from build123d import *

# Parameters (mm, degrees)
SKETCH1_R                       = 9.5
BOSS_EXTRUDE1_DEPTH             = 25
BOSS_EXTRUDE2_DEPTH             = 6
BOSS_EXTRUDE2_DEPTH_BACK        = 108
SKETCH2_R                       = 35
BOSS_EXTRUDE3_DEPTH             = 6.5
BOSS_EXTRUDE3_DEPTH_BACK        = 44.5
SKETCH3_R                       = 35
BOSS_EXTRUDE4_DEPTH             = 77
RIB1_REACH                      = 331.39
SKETCH5_WALLS_W                 = 19
SKETCH5_WALLS_H                 = 685.704980613
RIB2_REACH                      = 335.377
SKETCH6_WALLS_W                 = 19
SKETCH6_WALLS_H                 = 696.792690098
F_6_0MM_DOWEL_HOLE1_D           = 6
F_6_0MM_DOWEL_HOLE1_DEPTH       = 54
F_6_0MM_DOWEL_HOLE1_CSINK_D     = 6.05
F_6_0MM_DOWEL_HOLE1_CSINK_ANGLE = 90
F_6_0MM_DOWEL_HOLE1_TIP         = 1.802581857


with BuildPart() as part:
    # Sketch1 → Boss-Extrude1 (new body)
    with BuildSketch(Plane(origin=(0, 0, 0), x_dir=(1, 0, 0), z_dir=(0, 1, 0))):
        with BuildLine():
            Line((0, 102), (0, 0))
            Line((0, 0), (200, 0))
            Line((200, 0), (200, 213))
            Line((200, 213), (166, 213))
            Line((166, 213), (166, 147))
            ThreePointArc((166, 147), (152.819805153, 115.180194847), (121, 102))
            Line((121, 102), (0, 102))
        make_face()
        with Locations(Location((16, 57, 0), (0, 0, 270))):
            Circle(SKETCH1_R, mode=Mode.SUBTRACT)
        with Locations(Location((16, 19, 0), (0, 0, 270))):
            Circle(SKETCH1_R, mode=Mode.SUBTRACT)
        with Locations(Location((168, 19, 0), (0, 0, 270))):
            Circle(SKETCH1_R, mode=Mode.SUBTRACT)
        with Locations(Location((168, 57, 0), (0, 0, 270))):
            Circle(SKETCH1_R, mode=Mode.SUBTRACT)
    extrude(amount=BOSS_EXTRUDE1_DEPTH)



with BuildPart() as body_2:
    # Sketch2 → Boss-Extrude2 (new, two sides: drawn at the far end of the back side and taken through both)
    with BuildSketch(Plane.XY.offset(-BOSS_EXTRUDE2_DEPTH_BACK)):
        with Locations((83, 102)):
            Circle(SKETCH2_R)
    extrude(amount=BOSS_EXTRUDE2_DEPTH + BOSS_EXTRUDE2_DEPTH_BACK)


with BuildPart() as body_3:
    # Sketch3 → Boss-Extrude3 (new, two sides: drawn at the far end of the back side and taken through both)
    with BuildSketch(Plane(origin=(200, 0, 0), x_dir=(0, 0, -1), z_dir=(1, 0, 0)).offset(-BOSS_EXTRUDE3_DEPTH_BACK)):
        with Locations((188, 102)):
            Circle(SKETCH3_R)
    extrude(amount=BOSS_EXTRUDE3_DEPTH + BOSS_EXTRUDE3_DEPTH_BACK)


with BuildPart() as part_1:
    add(part.part)

    add(body_2.part)  # Boss-Extrude4 merges body 2

    add(body_3.part)  # Boss-Extrude4 merges body 3
    # Sketch4 → Boss-Extrude4 (add)
    with BuildSketch(Plane(origin=(0, 25, 0), x_dir=(1, 0, 0), z_dir=(0, 1, 0))):
        with BuildLine():
            Line((121, 102), (48, 102))
            Line((48, 102), (48, 83))
            Line((48, 83), (121, 83))
            ThreePointArc((121, 83), (166.254833996, 101.745166004), (185, 147))
            Line((185, 147), (185, 223))
            Line((185, 223), (166, 223))
            Line((166, 223), (166, 147))
            ThreePointArc((166, 147), (152.819805153, 115.180194847), (121, 102))
        make_face()
    extrude(amount=BOSS_EXTRUDE4_DEPTH)

    # Sketch5 walls → Rib1 (add, up to next)
    with BuildSketch(Plane(origin=(200, 0, 0), x_dir=(0, 0, -1), z_dir=(1, 0, 0)), mode=Mode.PRIVATE) as rib1_sk1:
        with Locations((188, 47.27733831)):
            Rectangle(SKETCH5_WALLS_W, SKETCH5_WALLS_H)
    rib1_tool1 = extrude(rib1_sk1.sketch, amount=-RIB1_REACH, mode=Mode.PRIVATE) - part_1.part
    add(rib1_tool1.solids().sort_by_distance((200, 47.277338311, -188))[0])

    # Sketch6 walls → Rib2 (add, up to next)
    with BuildSketch(Plane.XY, mode=Mode.PRIVATE) as rib2_sk1:
        with Locations((83, 44.133110569)):
            Rectangle(SKETCH6_WALLS_W, SKETCH6_WALLS_H)
    rib2_tool1 = extrude(rib2_sk1.sketch, amount=-RIB2_REACH, mode=Mode.PRIVATE) - part_1.part
    add(rib2_tool1.solids().sort_by_distance((83, 44.133110569, 0))[0])

    # Ø6.0mm Dowel Hole1
    with Locations(Plane(origin=(206.5, 99.319699539, -190.863289795), x_dir=(0, 0, 1), z_dir=(1, 0, 0))):
        with Locations((0, 0)):
            CounterSinkHole(F_6_0MM_DOWEL_HOLE1_D / 2, F_6_0MM_DOWEL_HOLE1_CSINK_D / 2, depth=F_6_0MM_DOWEL_HOLE1_DEPTH, counter_sink_angle=F_6_0MM_DOWEL_HOLE1_CSINK_ANGLE)
            with Locations((0, 0, -(F_6_0MM_DOWEL_HOLE1_DEPTH + F_6_0MM_DOWEL_HOLE1_TIP / 2))):  # 118° drill point
                Cone(0, F_6_0MM_DOWEL_HOLE1_D / 2, F_6_0MM_DOWEL_HOLE1_TIP, mode=Mode.SUBTRACT)


solid = part_1.part
Verification items for the finished model (mm, model axes). A direction names the side the tool comes from. Coordinates: 2 decimals unless noted, no trailing zeros. Loops run counter-clockwise (first coordinate to the right, second up) from the corner with the lowest first, then second, coordinate; pieces in that order, holes last. Notation, with made-up numbers: (86.5, -21) -> (132.5, -21) arc R35 cw to (132.5, 17) -> close; hole circle Ø9 at (5.5, 23.25). An arc over 180 degrees is marked (long way). Answer as a JSON object with one key per item and string values. Group by question number.
Item 1: Sectioned sample at D-D on y = 54. Record the boundary of the cut face in (x, z), plus the area to 3 significant figures.
Item 2: Tool access check on faces 1 (the flat face through (83, 102, -108)), 2 (the cylindrical face through (165.755, 62.961, -101.25)), 3 (the flat face through (183, 12, -213)), 4 (the flat face through (193, 46, -178.5)), 5 (the flat face through (185, 54, -210)). Record the directions out of +Z, -Z, +X, -X, +Y, -Y that give a thin tool (end or side, any length) a straight path to the whole face; none if there is none.
Item 3: Mould release check, pull along Y, two halves, no side actions. Record for faces 6 (the flat face through (36, 25, -52)), 7 (the cylindrical face through (12.361, 12.325, -48.224)), 8 (the flat face through (121, 0, -61)): +Y half, -Y half, draft (parallel to the pull), parting line (faces both ways), or undercut.
Item 4: Depth check by flat-ended pin: pin 1 (4 mm diameter, centred on y = 73, z = -48, fed in from -X); pin 2 (1 mm diameter, centred on x = 161, y = 53.5, fed in from +Z); pin 3 (16.5 mm diameter, centred on x = 194.5, y = 44.5, fed in from +Z); pin 4 (1 mm diameter, centred on x = 161, z = -58.5, fed in from +Y). Enter the tip coordinate at first touch or a pass-through.
Item 5: Sectioned sample at C-C on x = 16. Record the boundary of the cut face in (y, z).
Item 6: Scan lines: probe 1 along X at (y, z) = (13, -57); probe 2 along Y at (x, z) = (191, -9); probe 3 along X at (y, z) = (82, -204.5). Record each from-to range of solid material in increasing order.
Item 7: Sectioned sample at A-A on y = 9. Record the boundary of the cut face in (x, z), plus the area to 3 significant figures.
Item 8: Sectioned sample at B-B on z = -57. Record the boundary of the cut face in (x, y).
Evaluation:
{
 "1": {"outline": "(48, -102) -> (121, -102) arc R45 cw to (166, -147) -> (166, -223) -> (185, -223) -> (185, -197.5) -> (200, -197.5) -> (200, -178.5) -> (185, -178.5) -> (185, -147) arc R64 ccw to (121, -83) -> (92.5, -83) -> (92.5, 0) -> (73.5, 0) -> (73.5, -83) -> (48, -83) -> close", "area": "6,320 mm²"},
 "2": {"face 1": "-Z, -X, +Y, -Y", "face 2": "+Z, +X, +Y", "face 3": "-Z, +X, -X, -Y", "face 4": "+Z, +X", "face 5": "-Z, +X"},
 "3": {"face 6": "undercut", "face 7": "draft", "face 8": "-Y half"},
 "4": {"pin 1": "stops at x = 60.73", "pin 2": "stops at z = -96.64", "pin 3": "stops at z = -178.5", "pin 4": "passes through"},
 "5": {"outline": "(0, -102) -> (25, -102) -> (25, -66.5) -> (0, -66.5) -> close; (0, -47.5) -> (25, -47.5) -> (25, -28.5) -> (0, -28.5) -> close; (0, -9.5) -> (25, -9.5) -> (25, 0) -> (0, 0) -> close"},
 "6": {"probe 1": "x = 0 to 6.5, 25.5 to 158.5, 177.5 to 200", "probe 2": "y = 0 to 25", "probe 3": "x = 155.5 to 206.5"},
 "7": {"outline": "(0, -102) -> (121, -102) arc R45 cw to (166, -147) -> (166, -213) -> (200, -213) -> (200, 0) -> (0, 0) -> close; hole circle Ø19 at (16, -57); hole circle Ø19 at (16, -19); hole circle Ø19 at (168, -57); hole circle Ø19 at (168, -19)", "area": "23,500 mm²"},
 "8": {"outline": "(0, 0) -> (6.5, 0) -> (6.5, 25) -> (0, 25) -> close; (25.5, 0) -> (158.5, 0) -> (158.5, 25) -> (92.5, 25) -> (92.5, 68.31) arc R35 ccw (long way) to (73.5, 68.31) -> (73.5, 25) -> (25.5, 25) -> close; (177.5, 0) -> (200, 0) -> (200, 25) -> (177.5, 25) -> close"}
}
